The listing builds one solid part. Answer for the finished solid, in the listing's coordinates (mm). Face numbers are marked on the shaded views. A direction names the side the tool comes from. Round coordinates to 2 decimals unless told otherwise and drop trailing zeros. Order: outer loops, then holes, each group sorted by start corner. A loop starts at its lowest first (then second) coordinate and runs counter-clockwise, first axis right, second up. Notation, with made-up numbers: (64.5, 73) -> (114.5, 73) arc R23 ccw to (114.5, 103) -> close; hole circle Ø5 at (-34, 1.5). An arc over 180 degrees is marked (long way). Answer in a Markdown table with one row per item. Add a question column.
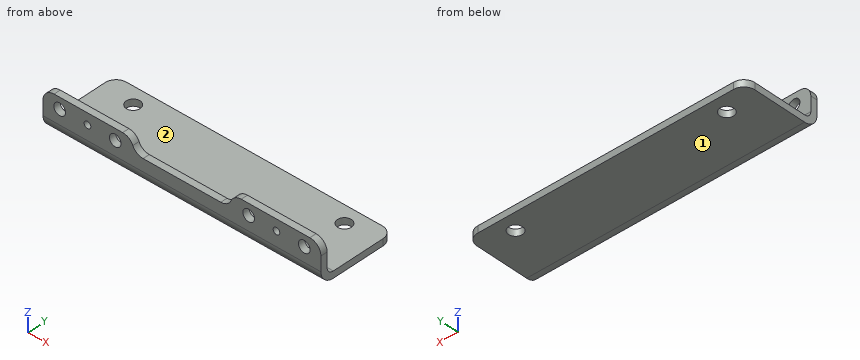
Autodesk Inventor part; units mm, degrees
ref_plane "YZ Plane" through (0, 0, 0) normal (1, 0, 0) x (0, 1, 0)
ref_plane "XZ Plane" through (0, 0, 0) normal (0, 1, 0) x (-1, 0, 0)
ref_plane "XY Plane" through (0, 0, 0) normal (0, 0, 1) x (1, 0, 0)
sketch "Эскиз1" plane through (0, 0, 0) normal (1, 0, 0) x (0, 1, 0)
  line L0 (-14, 0) -> (84, 0)
  line L1 (0, -7) -> (0, 42)
  line L2 (0, 35) -> (0, 0)
  line L3 (0, 0) -> (70, 0)
  line L4 (70, 6) -> (6, 6)
  line L5 (6, 6) -> (6, 35)
  line L6 (6, 35) -> (0, 35)
  line L7 (70, 6) -> (70, 0)
  dimension "d50" = 6
  dimension "d51" = 6
  dimension "d52" = 70
  dimension "d53" = 35
extrude "Выдавливание1" add sketch "Эскиз1" against normal blind 250
fillet "Сопряжение2" radius 6 1 edges at (-125, 6, 6)
fillet "Сопряжение3" radius 12 1 edges at (-125, 0, 0)
sketch "Эскиз5" plane through (-250, 0, 35) normal (0, -1, 0) x (1, 0, 0)
  line L0 (250, 0) -> (250, -23) construction
  line L1 (0, -23) -> (0, 0) construction
  line L2 (250, 0) -> (0, 0) construction
  line L3 (0, -10) -> (250, -10) construction
  circle A0 centre (15, -10) radius 5.25
  circle A1 centre (65, -10) radius 5.25
  circle A2 centre (235, -10) radius 5.25
  circle A3 centre (185, -10) radius 5.25
  point P0 (250, -35)
  dimension "d56" = 10
  dimension "d57" = 15
  dimension "d58" = 50
  dimension "d59" = 220
  dimension "d60" = 50
  dimension "d61" = 10.5
extrude "Выдавливание3" cut sketch "Эскиз5" against normal blind 10
fillet "Сопряжение4" radius 10 2 edges at (0, 3, 35) (-250, 3, 35)
sketch "Эскиз6" plane through (-250, 0, 12) normal (0, -1, 0) x (1, 0, 0)
  circle A0 centre (65, 13) radius 5.25 construction
  circle A1 centre (185, 13) radius 5.25 construction
  line L0 (240, 23) -> (10, 23) construction
  line L1 (80, 23) -> (80, 11)
  line L2 (80, 11) -> (170, 11)
  line L3 (170, 11) -> (170, 23)
  line L4 (80, 23) -> (170, 23)
  point P0 (250, -12)
  dimension "d65" = 15
  dimension "d66" = 15
  dimension "d67" = 12
extrude "Выдавливание4" cut sketch "Эскиз6" against normal blind 10
fillet "Сопряжение5" radius 10 4 edges at (-170, 3, 23) (-80, 3, 23) (-170, 3, 35) (-80, 3, 35)
fillet "Сопряжение6" radius 10 2 edges at (0, 70, 3) (-250, 70, 3)
sketch "Эскиз7" plane through (-250, 12, 6) normal (0, 0, 1) x (1, 0, 0)
  line L0 (240, -12) -> (178.3303, -12) construction
  circle A0 centre (220, 43) radius 6.25
  circle A1 centre (30, 43) radius 6.25
  line L1 (250, 48) -> (250, 0) construction
  line L2 (0, 0) -> (0, 48) construction
  point P0 (250, -12)
  dimension "d72" = 55
  dimension "d73" = 12.5
  dimension "d74" = 30
  dimension "d75" = 30
  dimension "d76" = 55
extrude "Выдавливание5" cut sketch "Эскиз7" against normal blind 10
sketch "Эскиз8" plane through (-250, 0, 12) normal (0, -1, 0) x (1, 0, 0)
  circle A0 centre (15, 13) radius 5.25 construction
  circle A1 centre (65, 13) radius 5.25 construction
  circle A2 centre (235, 13) radius 5.25 construction
  line L0 (15, 13) -> (65, 13) construction
  line L1 (185, 13) -> (235, 13) construction
  circle A3 centre (40, 13) radius 3
  circle A4 centre (210, 13) radius 3
  point P0 (250, -12)
  dimension "d79" = 25
  dimension "d80" = 6
  dimension "d81" = 6
  dimension "d82" = 25
extrude "Выдавливание6" cut sketch "Эскиз8" against normal blind 10
properties part number "ОПОРА_05"
Item 1: The part is cut by section D-D, the plane y = 38.5. Give the vertices of the cut face in (x, z), and give its area (3 significant figures).
Item 2: Find the intervals of material crossed by probe 1 along Y at (x, z) = (-80.5, 12.5); probe 2 along Z at (x, y) = (-15, 3), in increasing order. Write a range as [from, to].
Item 3: The part is cut by section B-B, the plane x = -220. Give the vertices of the cut face in (y, z), and give its area (3 significant figures).
Item 4: The part is cut by section C-C, the plane x = -141. Give the vertices of the cut face in (y, z).
Item 5: Flat-ended cylindrical pins translate along their axes: P1, Ø2, axis at x = -73.5, z = 17.5, coming from the -Y side; P2, Ø16, axis at x = -220, y = 55, coming from the +Z side; P3, Ø1.5, axis at x = -135.5, z = 9, coming from the -Y side; P4, Ø4, axis at x = -119.5, z = 20.5, coming from the +Y side. Find the tip coordinate at first contact, or state that the pin passes through.
Item 6: The part is cut by section A-A, the plane x = -15. Give the vertices of the cut face in (y, z), and give its area (3 significant figures).
Item 7: A tool of negligible diameter and unlimited length cuts with its end or side. For the marked faces 1 and 2, from which of +Z, -Z, +X, -X, +Y, -Y can it reach the whole face along a straight path? Write none if from no direction.
Resolved:
| question | item | result |
|---|---|---|
| 1 | outline | (-250, 0) -> (0, 0) -> (0, 6) -> (-250, 6) -> close |
| 1 | area | 1,500 mm2 |
| 2 | probe 1 | [0, 6] |
| 2 | probe 2 | [4.06, 19.75], [30.25, 35] |
| 3 | outline | (0, 12) arc R12 ccw to (12, 0) -> (48.75, 0) -> (48.75, 6) -> (12, 6) arc R6 cw to (6, 12) -> (6, 35) -> (0, 35) -> close; (61.25, 0) -> (70, 0) -> (70, 6) -> (61.25, 6) -> close |
| 3 | area | 496 mm2 |
| 4 | outline | (0, 12) arc R12 ccw to (12, 0) -> (70, 0) -> (70, 6) -> (12, 6) arc R6 cw to (6, 12) -> (6, 23) -> (0, 23) -> close |
| 5 | P1 | y = 0 |
| 5 | P2 | z = 6 |
| 5 | P3 | y = 0.21 |
| 5 | P4 | y = 6 |
| 6 | outline | (0, 12) arc R12 ccw to (12, 0) -> (70, 0) -> (70, 6) -> (12, 6) arc R6 cw to (6, 12) -> (6, 19.75) -> (0, 19.75) -> close; (0, 30.25) -> (6, 30.25) -> (6, 35) -> (0, 35) -> close |
| 6 | area | 508 mm2 |
| 7 | face 1 | -Z, +X, -X, +Y, -Y |
| 7 | face 2 | +Z, +X, -X, +Y |
